Design review of the part shown in the three views and the two pictorial views. Dimensions are in mm from the part's minimum x, y and z. A direction names the side the tool comes from. Coordinates: 2 decimals unless noted, no trailing zeros. Loops run counter-clockwise (first coordinate to the right, second up) from the corner with the lowest first, then second, coordinate; pieces in that order, holes last. Notation, with made-up numbers: (15, 29) -> (39, 29) arc R28 cw to (39, 62) -> close; hole circle Ø6 at (24.5, 61.25). An arc over 180 degrees is marked (long way). One line per item, written item: value.
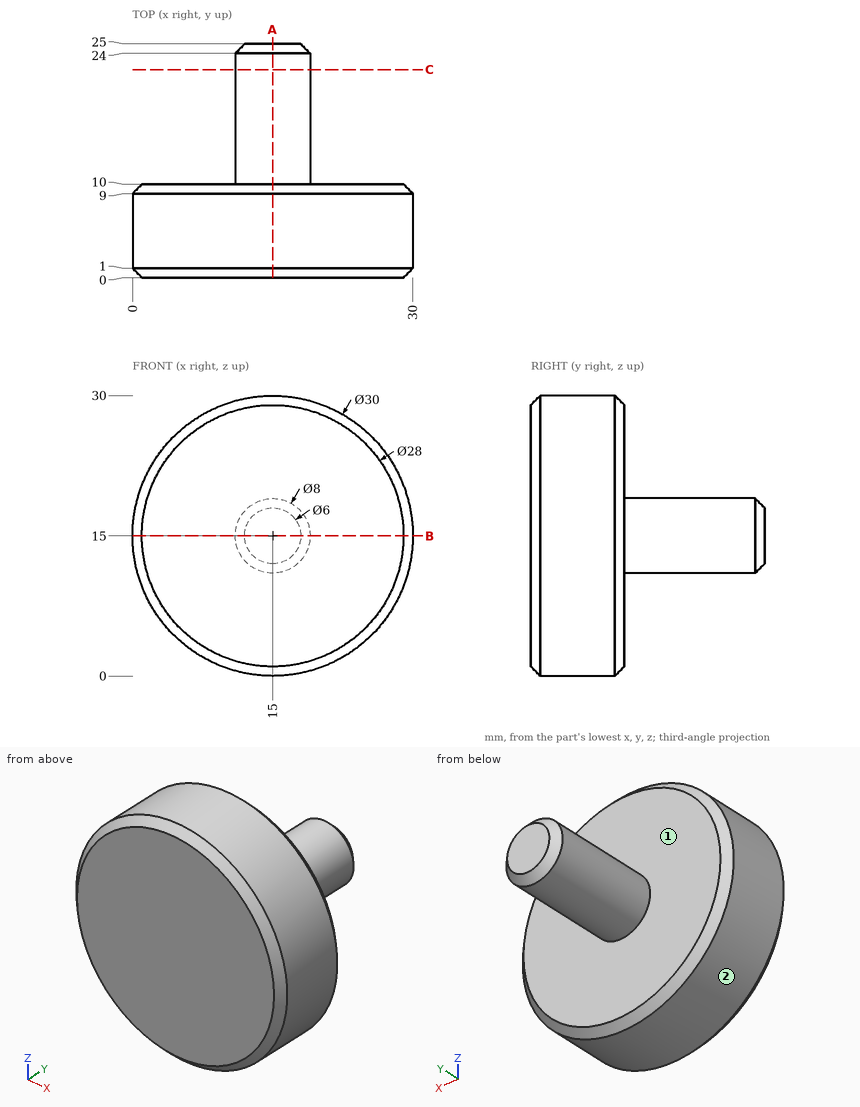
1. For the marked faces 1 and 2, list the 3-axis set-ups (+Z, -Z, +X, -X, +Y, -Y) from which the entire face can be reached by the end or side of a thin tool; tool diameter is ignored.
Return value:
face 1: +Y
face 2: +Y, -Y
2. Take a section at A-A, the plane x = 15. Give the boundary of the cut face in (y, z), and give its area (3 significant figures).
Return value:
outline: (0, 1) -> (1, 0) -> (9, 0) -> (10, 1) -> (10, 11) -> (24, 11) -> (25, 12) -> (25, 18) -> (24, 19) -> (10, 19) -> (10, 29) -> (9, 30) -> (1, 30) -> (0, 29) -> close
area: 417 mm2
3. To check wall thickness, follow probe 1 along Y at (x, z) = (9.25, 15); probe 2 along X at (y, z) = (16.25, 14.75); probe 3 along Z at (x, y) = (11.75, 23). State the ranges of each line that lie inside material, in increasing order. Write a range as from..to.
Return value:
probe 1: y = 0..10
probe 2: x = 11.01..18.99
probe 3: z = 12.67..17.33
4. Take a section at C-C, the plane y = 22.25. Give the boundary of the cut face in (x, z).
Return value:
outline: circle Ø8 at (15, 15)
5. Insertion check: pin 1 Ø8 at (x, z) = (15.5, 5.5) entering from +Y; pin 2 Ø2 at (x, y) = (9.5, 5) entering from -Z; pin 3 Ø2 at (y, z) = (13.5, 13) entering from +X. Each pin has a flat end and moves straight along its axis. Give the tip position at first contact, or say it passes through.
Return value:
pin 1: stops at y = 10
pin 2: stops at z = 0.69
pin 3: stops at x = 18.87
6. Take a section at B-B, the plane z = 15. Give the boundary of the cut face in (x, y), and give its area (3 significant figures).
Return value:
outline: (0, 1) -> (1, 0) -> (29, 0) -> (30, 1) -> (30, 9) -> (29, 10) -> (19, 10) -> (19, 24) -> (18, 25) -> (12, 25) -> (11, 24) -> (11, 10) -> (1, 10) -> (0, 9) -> close
area: 417 mm2
